from build123d import *

# Parameters (mm, degrees)
SKETCH1_W           = 55
SKETCH1_H           = 24
SKETCH1_R           = 3.75
BOSS_EXTRUDE1_DEPTH = 3
SKETCH3_W           = 4
SKETCH3_H           = 24
BOSS_EXTRUDE2_DEPTH = 24
SKETCH4_W           = 4
SKETCH4_H           = 24
BOSS_EXTRUDE3_DEPTH = 10
SKETCH5_R           = 1.55
CUT_EXTRUDE1_DEPTH  = 10
CUT_EXTRUDE2_REACH  = 48.111
SKETCH6_R           = 6.5
FILLET1_R           = 5


with BuildPart() as part:
    # Sketch1 → Boss-Extrude1 (new body)
    with BuildSketch(Plane.XY):
        Rectangle(SKETCH1_W, SKETCH1_H)
        with Locations((-19, -0.5)):
            Circle(SKETCH1_R, mode=Mode.SUBTRACT)
        with Locations((17, -0.5)):
            Circle(SKETCH1_R, mode=Mode.SUBTRACT)
    extrude(amount=BOSS_EXTRUDE1_DEPTH)

    # Sketch3 → Boss-Extrude2 (add)
    with BuildSketch(Plane.XY.offset(3)):
        with Locations((25.5, 0)):
            Rectangle(SKETCH3_W, SKETCH3_H)
    extrude(amount=BOSS_EXTRUDE2_DEPTH)

    # Sketch4 → Boss-Extrude3 (add)
    with BuildSketch(Plane(origin=(27.5, 0, 0), x_dir=(0, 0, -1), z_dir=(1, 0, 0))):
        with Locations((-25, 0)):
            Rectangle(SKETCH4_W, SKETCH4_H)
    extrude(amount=BOSS_EXTRUDE3_DEPTH)

    # Sketch5 → Cut-Extrude1 (cut)
    with BuildSketch(Plane.XY.offset(27)):
        with Locations((32.5, 7)):
            Circle(SKETCH5_R)
        with Locations((32.5, -0.5)):
            Circle(SKETCH5_R)
        with Locations((32.5, -8)):
            Circle(SKETCH5_R)
    extrude(amount=-CUT_EXTRUDE1_DEPTH, mode=Mode.SUBTRACT)

    # Sketch6 → Cut-Extrude2 (cut, up to next)
    with BuildSketch(Plane.XY.offset(3), mode=Mode.PRIVATE) as cut_extrude2_sk1:
        with Locations((-1.056622026, 12)):
            Circle(SKETCH6_R)
    cut_extrude2_tool1 = extrude(cut_extrude2_sk1.sketch, amount=-CUT_EXTRUDE2_REACH, mode=Mode.PRIVATE) & part.part
    # Sketch6 → Cut-Extrude2 (cut, up to next)
    with BuildSketch(Plane.XY.offset(3), mode=Mode.PRIVATE) as cut_extrude2_sk2:
        with Locations((-1.056622026, -12)):
            Circle(SKETCH6_R)
    cut_extrude2_tool2 = extrude(cut_extrude2_sk2.sketch, amount=-CUT_EXTRUDE2_REACH, mode=Mode.PRIVATE) & part.part
    add(cut_extrude2_tool1.solids().sort_by_distance((-1.056622, 12, 3))[0], mode=Mode.SUBTRACT)
    add(cut_extrude2_tool2.solids().sort_by_distance((-1.056622, -12, 3))[0], mode=Mode.SUBTRACT)

    # Fillet1
    fillet1_edges = [part.edges().sort_by_distance(p)[0] for p in [
        (23.5, 0, 27),
        (-27.5, 12, 1.5),
        (-27.5, -12, 1.5),
    ]]
    fillet(fillet1_edges, radius=FILLET1_R)


solid = part.part
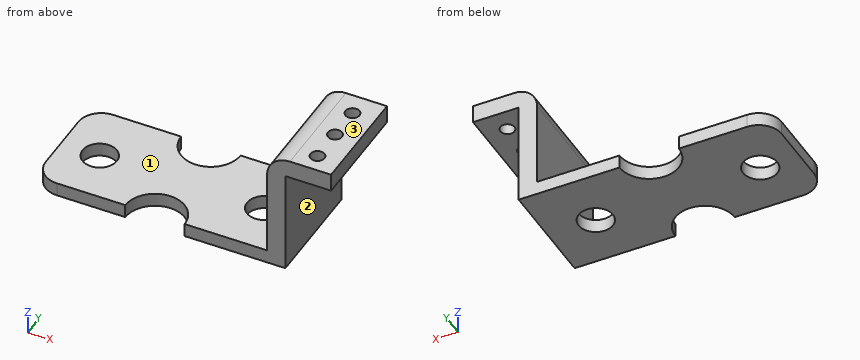
Check sheet for the modelled part. Datum: model origin and axes. Units: mm. Face numbers are marked on the shaded views. A direction names the side the tool comes from. Give positions to 0.01 mm unless a question says otherwise; leave off trailing zeros. Order: outer loops, then holes, each group sorted by start corner. A loop starts at its lowest first (then second) coordinate and runs counter-clockwise, first axis right, second up. Notation, with made-up numbers: M 79,55.5 L 125,55.5 A17 cw 125,64.5 Z; hole C -22.75,47 d5. An arc over 180 degrees is marked long. Answer as CSV lines item,"result". Start each with the question number.
Item 1: Cross-section at A-A on x = 32.5. Enter the section's corners in (y, z), plus the area to 3 significant figures.
Item 2: Cross-section at C-C on x = -19. Enter the section's corners in (y, z), plus the area to 3 significant figures.
Item 3: Cross-section at D-D on y = 0.25. Enter the section's corners in (x, z).
Item 4: Gauge pin test, flat ends, axial feed: P1, Ø2, axis at x = 16, y = 2.5, coming from the +Z side; P2, Ø11.5, axis at y = 5, z = 12, coming from the +X side; P3, Ø7, axis at x = 17, y = -0.5, coming from the -Z side; P4, Ø5, axis at x = 32.5, y = 7, coming from the -Z side. Record the tip position at first contact, or that the pin passes through.
Item 5: Thickness scan on line 1 (Y direction, x = 32.5, z = 23.95); line 2 (Y direction, x = -19, z = 0.85); line 3 (Z direction, x = 34, y = 10.75). Record the ranges inside material, lowest first. Write a range as [from, to].
Item 6: Cross-section at B-B on y = -8. Enter the section's corners in (x, z).
Item 7: Tool access check on the marked faces 1, 2 and 3. Record the directions out of +Z, -Z, +X, -X, +Y, -Y that give a thin tool (end or side, any length) a straight path to the whole face; none if there is none.
Established:
1,outline,"M -12,23 L -9.55,23 L -9.55,27 L -12,27 Z; M -6.45,23 L -2.05,23 L -2.05,27 L -6.45,27 Z; M 1.05,23 L 5.45,23 L 5.45,27 L 1.05,27 Z; M 8.55,23 L 12,23 L 12,27 L 8.55,27 Z"
1,area,"58.8 mm^2"
2,outline,"M -12,0 L -4.25,0 L -4.25,3 L -12,3 Z; M 3.25,0 L 12,0 L 12,3 L 3.25,3 Z"
2,area,"49.5 mm^2"
3,outline,"M -27.5,0 L -22.67,0 L -22.67,3 L -27.5,3 Z; M -15.33,0 L 13.33,0 L 13.33,3 L -15.33,3 Z; M 20.67,0 L 27.5,0 L 27.5,23 L 31.14,23 L 31.14,27 L 28.5,27 A5 ccw 23.5,22 L 23.5,3 L 20.67,3 Z; M 33.86,23 L 37.5,23 L 37.5,27 L 33.86,27 Z"
4,P1,"stops at z = 3"
4,P2,"stops at x = 27.5"
4,P3,"passes through"
4,P4,"stops at z = 23"
5,line 1,"y = [-12, -9.55], [-6.45, -2.05], [1.05, 5.45], [8.55, 12]"
5,line 2,"y = [-12, -4.25], [3.25, 12]"
5,line 3,"z = [23, 27]"
6,outline,"M -27.4,0 L -6.18,0 L -6.18,3 L -27.4,3 Z; M 4.07,0 L 27.5,0 L 27.5,23 L 30.95,23 L 30.95,27 L 28.5,27 A5 ccw 23.5,22 L 23.5,3 L 4.07,3 Z; M 34.05,23 L 37.5,23 L 37.5,27 L 34.05,27 Z"
7,face 1,"+Z, -X, +Y, -Y"
7,face 2,"-Z, +X, +Y, -Y"
7,face 3,"+Z, +X, -X, +Y, -Y"
